from build123d import *

# Parameters (mm, degrees)
SKETCH_1_R          = 2.5
EXTRUDE_1_DEPTH     = 10
FILLET_1_R          = 5
CUT_EXTRUDE_1_REACH = 85.254
SKETCH_2_R          = 2.5
CHAMFER_1_SIZE      = 10
CHAMFER_1_SIZE2     = 2.679491924


with BuildPart() as part:
    # 草圖1 → 填料-伸長1 (new body)
    with BuildSketch(Plane(origin=(0, 0, 0), x_dir=(0, 0, -1), z_dir=(1, 0, 0))):
        with BuildLine():
            Line((0, -7.5), (80.436404793, -7.5))
            Line((80.436404793, -7.5), (80.436404793, -3.535533906))
            ThreePointArc((80.436404793, -3.535533906), (78.971938699, 0), (80.436404793, 3.535533906))
            Line((80.436404793, 3.535533906), (80.436404793, 5))
            Line((80.436404793, 5), (3.436404793, 5))
            Line((3.436404793, 5), (-1.93911445, 19.003706397))
            Line((-1.93911445, 19.003706397), (-13.554844706, 14.544845311))
            Line((-13.554844706, 14.544845311), (-6.614588023, -3.535141479))
            ThreePointArc((-6.614588023, -3.535141479), (-3.85593302, -6.43286721), (0, -7.5))
        make_face()
        Circle(SKETCH_1_R, mode=Mode.SUBTRACT)
    extrude(amount=EXTRUDE_1_DEPTH)

    # 圓角1
    fillet_1_edges = [part.edges().sort_by_distance(p)[0] for p in [
        (5, 5, -3.436404793),
    ]]
    fillet(fillet_1_edges, radius=FILLET_1_R)

    # 草圖2 → 除料-伸長1 (cut, up to next)
    with BuildSketch(Plane.ZY, mode=Mode.PRIVATE) as cut_extrude_1_sk1:
        with Locations((7.632654751, 13.069153566)):
            Circle(SKETCH_2_R)
    cut_extrude_1_tool1 = extrude(cut_extrude_1_sk1.sketch, amount=-CUT_EXTRUDE_1_REACH, mode=Mode.PRIVATE) & part.part
    add(cut_extrude_1_tool1.solids().sort_by_distance((0, 13.069154, 7.632655))[0], mode=Mode.SUBTRACT)

    # 導角1
    chamfer_1_edges = [part.edges().sort_by_distance(p)[0] for p in [
        (5, -7.5, -80.436404793),
    ]]
    chamfer_1_side = [part.faces().sort_by_distance(p)[0] for p in [
        (5, -7.5, -40.218202397),
    ]]
    chamfer(chamfer_1_edges, length=CHAMFER_1_SIZE, length2=CHAMFER_1_SIZE2, reference=chamfer_1_side[0])


solid = part.part
Geometry check sheet. Reference: the model listing, model coordinates, mm. A direction names the side the tool comes from. Give positions to 0.01 mm unless a question says otherwise; leave off trailing zeros. Write each loop counter-clockwise with the first axis right and the second up, starting at its lowest first coordinate (ties: lowest second). Pieces come first, ordered by that corner, then holes. Notation, with made-up numbers: M -39.75,-7 L -9.75,-7 A17 ccw -9.75,-1 Z; hole C 10,54 d11. An arc over 180 degrees is marked long. Answer as CSV lines item,"result". Start each with the question number.
Q1. Release check for a two-part mould opening along Y. For faces 3 (the face through (5, -7.5, -35)), 4 (the face through (4.93, -0.055, -78.972)), 5 (the face through (10, 0, -33)), 6 (the face through (4.93, 11.548, 5.649)) record: pulls with the +Y half, pulls with the -Y half, needs draft (parallel to the pull), parting line crosses it, or undercut.
Q2. Go/stop test with flat-tipped pins: pin 1 (10 mm diameter, centred on y = 5, z = -30, fed in from -X); pin 2 (4 mm diameter, centred on y = 0, z = 0, fed in from +X); pin 3 (4 mm diameter, centred on x = 7, y = -0.5, fed in from +Z); pin 4 (3 mm diameter, centred on x = 2.5, z = -44.5, fed in from +Y). Record where each tip stops, or that it passes through.
Q3. Section check C-C, the plane x = 2.25. Record the cut outline in (y, z), then the cut area to 3 significant figures.
Q4. Section check D-D, the plane z = -8.5. Record the cut outline in (x, y), then the cut area to 3 significant figures.
Q5. Section check B-B, the plane z = 8. Record the cut outline in (x, y).
Q6. Material ranges on L1, parallel to Z at x = 5, y = 0.75; L2, parallel to Y at x = 5, z = -7; L3, parallel to Z at x = 9, y = -0.5, recorded low to high.
Q7. Tool access check on faces 1 (the face through (5, 5, -44)), 2 (the face through (0, 0, -33)). Record the directions out of +Z, -Z, +X, -X, +Y, -Y that give a thin tool (end or side, any length) a straight path to the whole face; none if there is none.
Q8. Section check A-A, the plane y = 0. Record the cut outline in (x, z).
Geometry says:
1,face 3,"pulls with the -Y half"
1,face 4,"undercut"
1,face 5,"needs draft"
1,face 6,"undercut"
2,pin 1,"x = 0"
2,pin 2,"through"
2,pin 3,"z = 8.55"
2,pin 4,"y = 5"
3,outline,"M -7.5,-70.44 L -4.82,-80.44 L -3.54,-80.44 A5 cw 3.54,-80.44 L 5,-80.44 L 5,-6.87 A5 cw 8.21,-2.2 L 19,1.94 L 14.54,13.55 L -3.54,6.61 A7.5 ccw -7.5,0 Z; hole C 0,0 d5; hole C 13.07,7.63 d5"
3,area,"1,190 mm^2"
4,outline,"M 0,-7.5 L 10,-7.5 L 10,5 L 0,5 Z"
4,area,"125 mm^2"
5,outline,"M 0,0.07 L 10,0.07 L 10,10.6 L 0,10.6 Z; M 0,15.54 L 10,15.54 L 10,16.68 L 0,16.68 Z"
6,L1,"-79.03 to -2.38, 2.38 to 8.26"
6,L2,"-7.5 to 5"
6,L3,"-79 to -2.45, 2.45 to 7.78"
7,face 1,"-Z, +X, -X, +Y"
7,face 2,"+Z, -Z, -X, +Y, -Y"
8,outline,"M 0,-78.97 L 10,-78.97 L 10,-2.5 L 0,-2.5 Z; M 0,2.5 L 10,2.5 L 10,7.97 L 0,7.97 Z"
